```python
from build123d import *

# Parameters (mm, degrees)
F1_DEPTH = 27.94
F2_R     = 8.120671
F3_DEPTH = 25.4


with BuildPart() as f1:
    # F0 (on Top) → F1 (new body)
    with BuildSketch(Plane.XY):
        Polygon((14.889965, 18.565336), (-46.177741, -34.020744), (14.889965, -34.020744), align=None)
    extrude(amount=-F1_DEPTH)

    # F2 (on face) → F3 (cut)
    with BuildSketch(Plane.YZ.offset(14.889965)):
        with Locations((-8.584474, -16.574016)):
            Circle(F2_R)
    extrude(amount=-F3_DEPTH, mode=Mode.SUBTRACT)


solid = f1.part
```
Model file for the job. Use its own axes, mm. Give positions to 0.01 mm unless a question says otherwise; leave off trailing zeros. Write each loop counter-clockwise with the first axis right and the second up, starting at its lowest first coordinate (ties: lowest second). Pieces come first, ordered by that corner, then holes. Notation, with made-up numbers: (16.5, 66) - (28.5, 66) arc R19 cw to (28.5, 81) - close; hole circle Ø7 at (-22.5, 73). An arc over 180 degrees is marked (long way). One line per question, with ' | ' between items. Start each with the question number.
(1) Slice it at B-B on y = -7.5. Write the cut outline in (x, z), plus the area to 3 significant figures.
(2) Slice it at C-C on x = 11. Write the cut outline in (y, z), plus the area to 3 significant figures.
(3) Two-plate mould, pull along Z, no slides. Class faces 1 (the face through (14.89, -8, -8)), 2 (the face through (-10.51, -10, -16)), 3 (the face through (2.368, -16.697, -16.217)), 4 (the face through (-3, -19, 0)): +Z half, -Z half, draft (parallel to the pull), parting line (faces both ways), or undercut.
(4) Slice it at D-D on z = -3. Write the cut outline in (x, y).
(5) Pin check, flat tips, straight feed: P1, Ø2, axis at x = 7, z = -17.5, coming from the +Y side; P2, Ø3, axis at x = -14, z = -12.5, coming from the +Y side; P3, Ø12, axis at y = -9.5, z = -18.5, coming from the -X side. Stop position of each tip, or through.
(6) Slice it at A-A on z = -21.5. Write the cut outline in (x, y), plus the area to 3 significant figures.
(7) Wall check: line 1 along Z through (x, y) = (-2, -9); line 2 along Y through (x, z) = (1, -22.5); line 3 along Y through (x, z) = (-13.5, -20). Give the ranges that are in metal, low to high. Write a range as from..to.
Results below:
1) outline: (-15.38, -27.94) - (14.89, -27.94) - (14.89, -24.62) - (-10.51, -24.62) - (-10.51, -8.53) - (14.89, -8.53) - (14.89, 0) - (-15.38, 0) - close | area: 437 mm^2
2) outline: (-34.02, -27.94) - (15.22, -27.94) - (15.22, 0) - (-34.02, 0) - close; hole circle Ø16.24 at (-8.58, -16.57) | area: 1,170 mm^2
3) face 1: draft | face 2: undercut | face 3: undercut | face 4: +Z half
4) outline: (-46.18, -34.02) - (14.89, -34.02) - (14.89, 18.57) - close
5) P1: y = 12.63 | P2: y = -5.02 | P3: x = -24.67
6) outline: (-46.18, -34.02) - (14.89, -34.02) - (14.89, -15.04) - (-10.51, -15.04) - (-10.51, -3.31) - close; (-9.14, -2.13) - (14.89, -2.13) - (14.89, 18.57) - close | area: 1,280 mm^2
7) line 1: -27.94..-24.68, -8.46..0 | line 2: -34.02..-14.14, -3.03..6.6 | line 3: -34.02..-5.88
